from build123d import *

# Parameters (mm, degrees)
SKETCH1_W                 = 18.85
SKETCH1_H                 = 6.28
BOSS_EXTRUDE1_DEPTH       = 8
SKETCH1_3_W               = 18.85
SKETCH1_3_H               = 6.28
BOSS_EXTRUDE2_DEPTH       = 8
BOSS_EXTRUDE3_DEPTH       = 8
SKETCH2_R                 = 2.75
SKETCH2_R_2               = 2.505012867
BOSS_EXTRUDE5_DEPTH       = 15
MIRROR2_COPY_1_SKETCH_R   = 2.75
MIRROR2_COPY_1_SKETCH_R_2 = 2.505012867
MIRROR2_COPY_1_DEPTH      = 15


with BuildPart() as part:
    # Sketch1 → Boss-Extrude1 (new body)
    with BuildSketch(Plane(origin=(0, 0, 0), x_dir=(1, 0, 0), z_dir=(0, 1, 0))):
        with Locations((-0.25472973, 1.292297297)):
            Rectangle(SKETCH1_W, SKETCH1_H)
    extrude(amount=BOSS_EXTRUDE1_DEPTH)



with BuildPart() as body_2:
    # Sketch1_3 → Boss-Extrude2 (new body)
    with BuildSketch(Plane(origin=(0, 0, 0), x_dir=(1, 0, 0), z_dir=(0, 1, 0))):
        with Locations((-0.25472973, 11.814937984)):
            Rectangle(SKETCH1_3_W, SKETCH1_3_H)
    extrude(amount=BOSS_EXTRUDE2_DEPTH)


with BuildPart() as part_1:
    add(part.part)

    add(body_2.part)  # Boss-Extrude3 merges body 2
    # Sketch1_5 → Boss-Extrude3 (add)
    with BuildSketch(Plane(origin=(0, 0, 0), x_dir=(1, 0, 0), z_dir=(0, 1, 0))):
        Polygon((-2.976050073, 6.553617641), (-2.376050073, 6.553617641), (-0.25472973, 8.674937984), (-0.85472973, 8.674937984), align=None)
        Polygon((-0.85472973, 4.432297297), (-0.25472973, 4.432297297), (-2.376050073, 6.553617641), (-2.976050073, 6.553617641), align=None)
        Polygon((-0.25472973, 8.674937984), (1.866590614, 6.553617641), (2.466590614, 6.553617641), (0.34527027, 8.674937984), align=None)
        Polygon((1.866590614, 6.553617641), (-0.25472973, 4.432297297), (0.34527027, 4.432297297), (2.466590614, 6.553617641), align=None)
    extrude(amount=BOSS_EXTRUDE3_DEPTH)

    # Sketch2 → Boss-Extrude5 (add)
    with BuildSketch(Plane(origin=(0, 0, 0), x_dir=(1, 0, 0), z_dir=(0, 1, 0))):
        with Locations((3.24527027, 11.814937984)):
            Circle(SKETCH2_R)
        with Locations((3.24527027, 11.814937984)):
            Circle(SKETCH2_R_2, mode=Mode.SUBTRACT)
    boss_extrude5 = extrude(amount=BOSS_EXTRUDE5_DEPTH)

    # Mirror1: Boss-Extrude5 across plane
    add(boss_extrude5.mirror(Plane(origin=(-0.25472973, 0, 0), x_dir=(0, 0, 1), z_dir=(1, 0, 0))))

    # Mirror2: Boss-Extrude5 across plane
    add(boss_extrude5.mirror(Plane(origin=(0, 0, -6.553617641), x_dir=(1, 0, 0), z_dir=(0, 0, -1))))

    # Mirror2 copy 1 sketch → Mirror2 copy 1 (add)
    with BuildSketch(Plane(origin=(-0.509459459, 0, -13.107235282), x_dir=(-1, 0, 0), z_dir=(0, 1, 0))):
        with Locations((3.24527027, 11.814937984)):
            Circle(MIRROR2_COPY_1_SKETCH_R)
        with Locations((3.24527027, 11.814937984)):
            Circle(MIRROR2_COPY_1_SKETCH_R_2, mode=Mode.SUBTRACT)
    extrude(amount=MIRROR2_COPY_1_DEPTH)


solid = part_1.part
Can you work these out from the model? Positions are in its coordinate system, mm. A direction names the side the tool comes from. Round coordinates to 2 decimals unless told otherwise and drop trailing zeros. Write each loop counter-clockwise with the first axis right and the second up, starting at its lowest first coordinate (ties: lowest second). Pieces come first, ordered by that corner, then holes. Notation, with made-up numbers: M 33.25,18 L 62.25,18 A23 ccw 62.25,38 Z; hole C 67,-11 d9. An arc over 180 degrees is marked long. Use a Markdown table: item, result.
Item 1: I want a section at C-C (y = 4.75). List the corners of the cut face in (x, z) for me.
Found:
| item | result |
|---|---|
| outline | M -9.68,-14.95 L 9.17,-14.95 L 9.17,-8.67 L 0.35,-8.67 L 2.47,-6.55 L 0.35,-4.43 L 9.17,-4.43 L 9.17,1.85 L -9.68,1.85 L -9.68,-4.43 L -0.85,-4.43 L -2.98,-6.55 L -0.85,-8.67 L -9.68,-8.67 Z; hole M -2.38,-6.55 L -0.25,-8.67 L 1.87,-6.55 L -0.25,-4.43 Z |
Item 2: For pin 1 Ø4 at (x, y) = (-5.5, 11) entering from -Z; pin 2 Ø4.5 at (x, z) = (3.25, -11.81) entering from +Y; pin 3 Ø4 at (x, y) = (-4.5, 13.5) entering from +Z, each with a flat end and sliding along its axis, tell me the tip position at first contact or that it passes through.
Found:
| item | result |
|---|---|
| pin 1 | stops at z = -14.56 |
| pin 2 | stops at y = 8 |
| pin 3 | stops at z = 1.46 |
Item 3: We'd pull the mould along X, two halves only. Please class faces 6 (the face through (5, 4, -4.432)), 7 (the face through (3, 8, -1)), 8 (the face through (1.391, 3.944, -5.478)): released by +X, released by -X, zero draft, split by the parting line, or undercut.
Found:
| item | result |
|---|---|
| face 6 | zero draft |
| face 7 | undercut |
| face 8 | released by +X |
Item 4: I want a section at D-D (z = -3). List the corners of the cut face in (x, y) for me, and give its area (3 significant figures).
Found:
| item | result |
|---|---|
| outline | M -9.68,0 L 9.17,0 L 9.17,8 L 5.4,8 L 5.4,15 L 5.08,15 L 5.08,8 L 1.41,8 L 1.41,15 L 1.09,15 L 1.09,8 L -1.6,8 L -1.6,15 L -1.92,15 L -1.92,8 L -5.59,8 L -5.59,15 L -5.91,15 L -5.91,8 L -9.68,8 Z |
| area | 160 mm2 |
Item 5: I want a section at B-B (y = 11.5). List the corners of the cut face in (x, z) for me, and give its area (3 significant figures).
Found:
| item | result |
|---|---|
| outline | C -3.75,-11.81 d5.5; C -3.75,-1.29 d5.5; C 3.25,-11.81 d5.5; C 3.25,-1.29 d5.5; hole C -3.75,-11.81 d5.01; hole C -3.75,-1.29 d5.01; hole C 3.25,-11.81 d5.01; hole C 3.25,-1.29 d5.01 |
| area | 16.2 mm2 |
Item 6: Which directions (+Z, -Z, +X, -X, +Y, -Y) give clear straight access to the entire face, cutting with the end or side of a thin tool? Please do faces 1 (the face through (1.42, 3.94, -7.6)), 2 (the face through (-1.6, 11.5, -3)), 3 (the face through (0.79, 3.94, -7.63)), 4 (the face through (-9.68, 4, -1)), 5 (the face through (-1.93, 3.94, -5.51)).
Found:
| item | result |
|---|---|
| face 1 | +X, +Y, -Y |
| face 2 | +Y |
| face 3 | +Y, -Y |
| face 4 | +Z, -Z, -X, +Y, -Y |
| face 5 | -X, +Y, -Y |
Item 7: I want a section at A-A (x = 8.25). List the corners of the cut face in (y, z) for me, and give its area (3 significant figures).
Found:
| item | result |
|---|---|
| outline | M 0,-14.95 L 8,-14.95 L 8,-8.67 L 0,-8.67 Z; M 0,-4.43 L 8,-4.43 L 8,1.85 L 0,1.85 Z |
| area | 100 mm2 |
Item 8: If I drill on line 1 along Z through (x, y) = (4.25, 4.75); line 2 along Z through (x, y) = (-4, 12.75); line 3 along Z through (x, y) = (1, 10), over which ranges is the centre line in solid material (lowest first)? Write a range as [from, to].
Found:
| item | result |
|---|---|
| line 1 | z = [-14.95, -8.67], [-4.43, 1.85] |
| line 2 | z = [-14.55, -14.31], [-9.32, -9.08], [-4.03, -3.79], [1.2, 1.45] |
| line 3 | z = [-13.4, -12.93], [-10.7, -10.23], [-2.88, -2.4], [-0.18, 0.3] |
